Design review of the part built by this model. Coordinates are the model's own, in mm. A direction names the side the tool comes from. Round coordinates to 2 decimals unless told otherwise and drop trailing zeros. Write each loop counter-clockwise with the first axis right and the second up, starting at its lowest first coordinate (ties: lowest second). Pieces come first, ordered by that corner, then holes. Notation, with made-up numbers: (60, 41.25) -> (111, 41.25) arc R16 ccw to (111, 61.25) -> close; hole circle Ø10 at (58.5, 44). An arc over 180 degrees is marked (long way). One line per question, with ' | ' between items. Start each with the question number.
1) Consider section A-A (x = -82.5). Give the boundary of the cut face in (y, z) (3 decimals).
2) Insertion check: pin 1 Ø8 at (x, z) = (-71, 22) entering from +Y; pin 2 Ø4 at (x, y) = (-3.5, 69) entering from +Z; pin 3 Ø3.5 at (y, z) = (75, 26.5) entering from -X; pin 4 Ø2.5 at (y, z) = (75, 27) entering from -X. Each pin has a flat end and moves straight along its axis. Give the tip position at first contact, or say it passes through.
3) Consider section B-B (y = 30). Give the boundary of the cut face in (x, z), then the cut area to 3 significant figures.
4) For faces 4 (the flat face through (-30.17, -2.97, 18.73)), 5 (the flat face through (-54, 72.5, 19)), 6 (the flat face through (-4, 69, 2)), 7 (the flat face through (-27.25, 75, 19)), list the 3-axis set-ups (+Z, -Z, +X, -X, +Y, -Y) from which the entire face can be reached by the end or side of a thin tool; tool diameter is ignored.
5) Consider section C-C (y = 60). Give the boundary of the cut face in (x, z).
6) Consider section D-D (z = 13.5). Count the separate pieces of the cut face and the enclosed holes in it, then the cut area to 3 significant figures.
7) For probe 1 along Y at (x, z) = (-23.5, 4); probe 2 along X at (y, z) = (4, 16.75); probe 3 along Y at (x, z) = (-102.5, 25.25), list the stretches that pass through material, from the lowest coordinate up.
8) Mouldability with a two-part tool opening along X and no side actions: class faces 1 (the flat face through (-82, -4.5, 19)), 2 (the flat face through (-24, -6, 19)), 3 (the flat face through (-87.876, -3.39, 18.734)) as +X half, -X half, draft (parallel to the pull), parting line (faces both ways), or undercut.
```python
from build123d import *

# Parameters (mm, degrees)
F0_W      = 106.5
F0_H      = 72.5
F1_DEPTH  = 38
F2_T      = -2
F3_W      = 6
F3_H      = 3
F4_DEPTH  = 38
F5_R      = 2
F6_R      = 4
F7_DEPTH  = 2
F8_R      = 2.75
F8_R_2    = 2
F9_DEPTH  = 30
F10_W     = 105
F10_H     = 71.125
F10_W_2   = 103.5
F10_H_2   = 69.625
F11_DEPTH = 1.5


with BuildPart() as f1:
    # F0 (on Top) → F1 (new body)
    with BuildSketch(Plane.XY):
        with Locations((-53.25, 36.25)):
            Rectangle(F0_W, F0_H)
    extrude(amount=F1_DEPTH)

    # F2
    f2_openings = [f1.faces().sort_by_distance(p)[0] for p in [
        (-53.25, 36.25, 38),
    ]]
    offset(amount=F2_T, openings=f2_openings)

    # F3 (on Top) → F4 (join)
    with BuildSketch(Plane.XY):
        Polygon((-28.048755, 78.5), (-32.25, 72.5), (-16.25, 72.5), (-20.451245, 78.5), align=None)
        with Locations((-24.25, 75.5)):
            Rectangle(F3_W, F3_H, mode=Mode.SUBTRACT)
        Polygon((-74.25, 72.5), (-78.451245, 78.5), (-86.048755, 78.5), (-90.25, 72.5), align=None)
        with Locations((-82.25, 75.5)):
            Rectangle(F3_W, F3_H, mode=Mode.SUBTRACT)
        Polygon((-74.25, 0), (-90.25, 0), (-86.048755, -6), (-78.451245, -6), align=None)
        with Locations((-82.25, -3)):
            Rectangle(F3_W, F3_H, mode=Mode.SUBTRACT)
        Polygon((-32.25, 0), (-28.048755, -6), (-20.451245, -6), (-16.25, 0), align=None)
        with Locations((-24.25, -3)):
            Rectangle(F3_W, F3_H, mode=Mode.SUBTRACT)
    extrude(amount=F4_DEPTH)

    # F5
    f5_edges = [f1.edges().sort_by_distance(p)[0] for p in [
        (-86.048755, 78.5, 19),
        (-78.451245, 78.5, 19),
        (-74.25, 72.5, 19),
        (-90.25, 72.5, 19),
        (-32.25, 72.5, 19),
        (-28.048755, 78.5, 19),
        (-20.451245, 78.5, 19),
        (-16.25, 72.5, 19),
        (-74.25, 0, 19),
        (-78.451245, -6, 19),
        (-90.25, 0, 19),
        (-32.25, 0, 19),
        (-28.048755, -6, 19),
        (-20.451245, -6, 19),
        (-16.25, 0, 19),
    ]]
    fillet(f5_edges, radius=F5_R)

    # F6 (on face) → F7 (cut, through all)
    with BuildSketch(Plane(origin=(-106.5, 0, 0), x_dir=(0, -1, 0), z_dir=(-1, 0, 0))):
        with Locations((-58, 6)):
            Circle(F6_R)
    extrude(amount=-F7_DEPTH, mode=Mode.SUBTRACT)

    # F8 (on face) → F9 (join)
    with BuildSketch(Plane.XY.offset(2)):
        with Locations((-102.5, 68.5)):
            Circle(F8_R)
        with Locations((-102.5, 68.5)):
            Circle(F8_R_2, mode=Mode.SUBTRACT)
        with Locations((-4, 68.5)):
            Circle(F8_R)
        with Locations((-4, 68.5)):
            Circle(F8_R_2, mode=Mode.SUBTRACT)
        with Locations((-4, 4)):
            Circle(F8_R)
        with Locations((-4, 4)):
            Circle(F8_R_2, mode=Mode.SUBTRACT)
        with Locations((-102.5, 4)):
            Circle(F8_R)
        with Locations((-102.5, 4)):
            Circle(F8_R_2, mode=Mode.SUBTRACT)
    extrude(amount=F9_DEPTH)

    # F10 (on face) → F11 (cut)
    with BuildSketch(Plane.XY.offset(38)):
        with Locations((-53.25, 36.3125)):
            Rectangle(F10_W, F10_H)
        with Locations((-53.25, 36.3125)):
            Rectangle(F10_W_2, F10_H_2, mode=Mode.SUBTRACT)
    extrude(amount=-F11_DEPTH, mode=Mode.SUBTRACT)


solid = f1.part
```
From the geometry:
1) outline: (-6, 0) -> (-4.5, 0) -> (-4.5, 38) -> (-6, 38) -> close; (-1.5, 0) -> (74, 0) -> (74, 38) -> (71.875, 38) -> (71.875, 36.5) -> (71.125, 36.5) -> (71.125, 38) -> (70.5, 38) -> (70.5, 2) -> (2, 2) -> (2, 38) -> (1.5, 38) -> (1.5, 36.5) -> (0.75, 36.5) -> (0.75, 38) -> (-1.5, 38) -> close; (77, 0) -> (78.5, 0) -> (78.5, 38) -> (77, 38) -> close
2) pin 1: stops at y = 73.57 | pin 2: stops at z = 38 | pin 3: stops at x = -89.73 | pin 4: stops at x = -89.37
3) outline: (-106.5, 0) -> (0, 0) -> (0, 38) -> (-0.75, 38) -> (-0.75, 36.5) -> (-1.5, 36.5) -> (-1.5, 38) -> (-2, 38) -> (-2, 2) -> (-104.5, 2) -> (-104.5, 38) -> (-105, 38) -> (-105, 36.5) -> (-105.75, 36.5) -> (-105.75, 38) -> (-106.5, 38) -> close | area: 355 mm2
4) face 4: +Z, -Z, -Y | face 5: +Z, -Z, +Y | face 6: +Z | face 7: +Z, -Z
5) outline: (-106.5, 0) -> (0, 0) -> (0, 38) -> (-0.75, 38) -> (-0.75, 36.5) -> (-1.5, 36.5) -> (-1.5, 38) -> (-2, 38) -> (-2, 2) -> (-104.5, 2) -> (-104.5, 2.54) -> (-106.5, 2.54) -> close; (-106.5, 9.46) -> (-104.5, 9.46) -> (-104.5, 38) -> (-105, 38) -> (-105, 36.5) -> (-105.75, 36.5) -> (-105.75, 38) -> (-106.5, 38) -> close
6) separate pieces: 1 | enclosed holes: 13 | area: 941 mm2
7) probe 1: y = -6 to -4.5, -1.5 to 2, 70.5 to 74, 77 to 78.5 | probe 2: x = -106.5 to -104.5, -100.5 to -99.75, -6.75 to -6, -2 to 0 | probe 3: y = 0 to 2, 6 to 6.75, 65.75 to 66.5, 70.5 to 72.5
8) face 1: undercut | face 2: draft | face 3: -X half
